```python
from build123d import *

# Parameters (mm, degrees)
F0_R     = 19
F0_R_2   = 16
F1_DEPTH = 4
F2_W     = 6
F2_H     = 3
F3_DEPTH = 27
F5_DEPTH = 4
F6_D     = 3.3
F6_DEPTH = 7
F6_TIP   = 0.9914200214


with BuildPart() as f1:
    # F0 (on Right) → F1 (new body, symmetric)
    with BuildSketch(Plane.YZ):
        Circle(F0_R)
        Circle(F0_R_2, mode=Mode.SUBTRACT)
    extrude(amount=F1_DEPTH, both=True)

    # F2 (on Front) → F3 (join, symmetric)
    with BuildSketch(Plane.XZ):
        with Locations((-1, 0)):
            Rectangle(F2_W, F2_H)
    extrude(amount=F3_DEPTH, both=True)

    # F0 (on Right) → F5 (cut, symmetric)
    with BuildSketch(Plane.YZ):
        Circle(F0_R_2)
    extrude(amount=F5_DEPTH, both=True, mode=Mode.SUBTRACT)

    # F6
    with Locations(Plane.XY.offset(1.5)):
        with Locations((-1, 24), (-1, -24)):
            Hole(F6_D / 2, depth=F6_DEPTH)
            with Locations((0, 0, -(F6_DEPTH + F6_TIP / 2))):  # 118° drill point
                Cone(0, F6_D / 2, F6_TIP, mode=Mode.SUBTRACT)


solid = f1.part
```
Source: CAD feature listing. Evaluate the final solid. Frame: model axes, mm. A direction names the side the tool comes from. Round coordinates to 2 decimals unless told otherwise and drop trailing zeros. Write each loop counter-clockwise with the first axis right and the second up, starting at its lowest first coordinate (ties: lowest second). Pieces come first, ordered by that corner, then holes. Notation, with made-up numbers: M 57.5,77 L 61.5,77 A10 cw 61.5,88 Z; hole C -12,51 d10. An arc over 180 degrees is marked long. Answer as a JSON object with one key per item and string values. Group by question number.
(1) Reachability of faces 1 (the flat face through (2, 23, 0)), 2 (the flat face through (-1, -22, 1.5)), 3 (the flat face through (-1, -22, -1.5)) from +Z, -Z, +X, -X, +Y, -Y: full face, straight path, thin tool, end or side. Return the list, or none.
(2) Section query B-B on y = 24. Output: boundary loops of the cut face in (x, z).
(3) Section query C-C on x = -1. Output: boundary loops of the cut face in (y, z).
(4) First-contact query: pin 1 (2 mm diameter, centred on x = 2, z = -4, fed in from +Y); pin 2 (3 mm diameter, centred on x = -1, y = -24, fed in from +Z); pin 3 (2.5 mm diameter, centred on y = 23, z = -0.5, fed in from +X); pin 4 (1.5 mm diameter, centred on x = -1.5, y = -13.5, fed in from +Z). Flat tips, straight axial feed; report the tip coordinate or a pass-through.
(5) Mould query, pull axis Y, two halves, no side actions, for faces 4 (the flat face through (-1, 22, -1.5)), 5 (the cylindrical face through (-0.785, 25.636, -0.021)), 6 (the flat face through (-1, -27, 0)). Classes: +Y half, -Y half, draft (parallel to the pull), parting line (faces both ways), or undercut.
(6) Section query A-A on z = 0. Output: boundary loops of the cut face in (x, y).
(7) Ray query, line 1 (Y direction, x = -1, z = -0.4) (3 decimals); line 2 (Z direction, x = -2.5, y = -0.5); line 3 (Y direction, x = -1.25, z = 12.5). Return the intervals inside material, ascending. Write a range as [from, to].
(8) Section query D-D on z = -12. Output: boundary loops of the cut face in (x, y).
Computed values:
{
 "1": {"face 1": "+Z, -Z, +X, +Y", "face 2": "+Z, +X, -X, -Y", "face 3": "-Z, +X, -X, -Y"},
 "2": {"outline": "M -4,-1.5 L -2.65,-1.5 L -2.65,1.5 L -4,1.5 Z; M 0.65,-1.5 L 2,-1.5 L 2,1.5 L 0.65,1.5 Z"},
 "3": {"outline": "M -27,-1.5 L -25.65,-1.5 L -25.65,1.5 L -27,1.5 Z; M -22.35,-1.5 L -18.94,-1.5 A19 ccw 18.94,-1.5 L 22.35,-1.5 L 22.35,1.5 L 18.94,1.5 A19 ccw -18.94,1.5 L -22.35,1.5 Z; M 25.65,-1.5 L 27,-1.5 L 27,1.5 L 25.65,1.5 Z; hole C 0,0 d32"},
 "4": {"pin 1": "y = 18.76", "pin 2": "through", "pin 3": "x = 2", "pin 4": "z = 14.09"},
 "5": {"face 4": "draft", "face 5": "undercut", "face 6": "-Y half"},
 "6": {"outline": "M -4,-27 L 2,-27 L 2,-19 L 4,-19 L 4,-16 L -4,-16 Z; M -4,16 L 4,16 L 4,19 L 2,19 L 2,27 L -4,27 Z; hole C -1,-24 d3.3; hole C -1,24 d3.3"},
 "7": {"line 1": "[-27, -25.65], [-22.35, -15.995], [15.995, 22.35], [25.65, 27]", "line 2": "[-18.99, -15.99], [15.99, 18.99]", "line 3": "[-14.31, -9.99], [9.99, 14.31]"},
 "8": {"outline": "M -4,-14.73 L 4,-14.73 L 4,-10.58 L -4,-10.58 Z; M -4,10.58 L 4,10.58 L 4,14.73 L -4,14.73 Z"}
}
